Geometry check sheet. Reference: the model listing, model coordinates, mm. Coordinates: 2 decimals unless noted, no trailing zeros. Loops run counter-clockwise (first coordinate to the right, second up) from the corner with the lowest first, then second, coordinate; pieces in that order, holes last.
Autodesk Inventor part; units mm, degrees
ref_plane "YZ Plane" through (0, 0, 0) normal (1, 0, 0) x (0, 1, 0)
ref_plane "XZ Plane" through (0, 0, 0) normal (0, 1, 0) x (-1, 0, 0)
ref_plane "XY Plane" through (0, 0, 0) normal (0, 0, 1) x (1, 0, 0)
ref_plane "Work Plane1" through (0, 0, 0) normal (0, 0, 1) x (1, 0, 0)
sketch "Sketch1" plane through (0, 0, 0) normal (0, 0, 1) x (1, 0, 0)
  circle A0 centre (-16.4512, 11.8299) radius 1.45
  circle A1 centre (-37.2, 11.8299) radius 1.45
  line L0 (-41.2012, 5.1624) -> (-41.2012, -2.0876)
  line L1 (-41.2012, -2.0876) -> (-38.2, -2.0876)
  line L2 (-38.2, -2.0876) -> (-38.2, -7.0876)
  line L3 (-38.2, -7.0876) -> (-41.2, -7.0876)
  line L4 (-41.2, -7.0876) -> (-41.2, -48.1342)
  line L5 (-41.2, -48.1342) -> (-20.7938, -54.7646)
  line L6 (-20.7938, -54.7646) -> (28.3237, 8.1029)
  line L7 (28.3237, 8.1029) -> (54.2162, 8.1029)
  line L8 (54.2162, 8.1029) -> (54.2162, 31.454)
  line L9 (54.2162, 31.454) -> (27.1735, 40.2407)
  line L10 (27.1735, 40.2407) -> (-12.4512, -10.4765)
  line L11 (-12.4512, -10.4765) -> (-12.4512, 5.6624)
  line L12 (-12.4512, 5.6624) -> (-15.7012, 5.6624)
  line L13 (-15.7012, 5.6624) -> (-15.7012, 8.1624)
  line L14 (-15.7012, 8.1624) -> (-12.4512, 8.1624)
  line L15 (-12.4512, 8.1624) -> (-12.4512, 32.1624)
  line L16 (-31.5338, 32.1624) -> (-41.2, 32.1624)
  line L17 (-41.2, 32.1624) -> (-41.2, 8.1624)
  line L18 (-41.2, 8.1624) -> (-38.2, 8.1624)
  line L19 (-38.2, 8.1624) -> (-38.2, 5.6624)
  line L20 (-38.2, 5.6624) -> (-41.2, 5.6624)
  line L21 (-41.2, 5.6624) -> (-41.2, 5.1624)
  line L22 (-41.2, 5.1624) -> (-41.2012, 5.1624)
  line L23 (-12.7012, -2.0876) -> (-12.7012, -7.0876)
  line L24 (-12.7012, -7.0876) -> (-15.7012, -7.0876)
  line L25 (-15.7012, -7.0876) -> (-15.7012, -2.0876)
  line L26 (-15.7012, -2.0876) -> (-12.7012, -2.0876)
  line L27 (-16.239, -63.6047) -> (29.7869, 5.1029)
  line L28 (29.7869, 5.1029) -> (60.3683, 5.1029)
  line L29 (60.3683, 5.1029) -> (60.3683, 31.9539)
  line L30 (60.3683, 31.9539) -> (57.3683, 35.6787)
  line L31 (57.3683, 35.6787) -> (27.4078, 45.4135)
  line L32 (27.4078, 45.4135) -> (-9.4512, -1.7639)
  line L33 (-9.4512, -1.7639) -> (-9.4512, 35.1624)
  line L34 (-9.4512, 35.1624) -> (-42.2, 35.1624)
  line L35 (-42.2, 35.1624) -> (-44.2, 35.1624)
  line L36 (-44.2, 35.1624) -> (-44.2, -54.5196)
  line L37 (-44.2, -54.5196) -> (-16.239, -63.6047)
  line L38 (-41.2, 5.1624) -> (-41.2, 5.6624)
  line L39 (-41.2, 5.6624) -> (-38.2, 5.6624)
  line L40 (-38.2, 5.6624) -> (-38.2, 8.1624)
  line L41 (-38.2, 8.1624) -> (-41.2, 8.1624)
  line L42 (-41.2, 8.1624) -> (-41.2, 32.1624)
  line L43 (-41.2, 32.1624) -> (-12.4512, 32.1624)
  line L44 (-12.4512, 32.1624) -> (-12.4512, 8.1624)
  line L45 (-12.4512, 8.1624) -> (-15.7012, 8.1624)
  line L46 (-15.7012, 8.1624) -> (-15.7012, 5.6624)
  line L47 (-15.7012, 5.6624) -> (-12.4512, 5.6624)
  line L48 (-12.4512, 5.6624) -> (-12.4512, -10.4765)
  line L49 (-12.4512, -10.4765) -> (27.1735, 40.2407)
  line L50 (27.1735, 40.2407) -> (54.2162, 31.454)
  line L51 (54.2162, 31.454) -> (54.2162, 8.1029)
  line L52 (54.2162, 8.1029) -> (28.3237, 8.1029)
  line L53 (28.3237, 8.1029) -> (-20.7938, -54.7646)
  line L54 (-20.7938, -54.7646) -> (-41.2, -48.1342)
  line L55 (-41.2, -48.1342) -> (-41.2, -7.0876)
  line L56 (-41.2, -7.0876) -> (-38.2, -7.0876)
  line L57 (-38.2, -7.0876) -> (-38.2, -2.0876)
  line L58 (-38.2, -2.0876) -> (-41.2012, -2.0876)
  line L59 (-41.2012, -2.0876) -> (-41.2012, 5.1624)
  line L60 (-41.2012, 5.1624) -> (-41.2, 5.1624)
  circle A2 centre (43.9499, 17.9141) radius 1.4
  circle A3 centre (43.9499, 30.4141) radius 1.4
  line L61 (-31.5338, 25.1624) -> (-31.5338, 32.1624)
  line L62 (-12.4512, 32.1624) -> (-22.3686, 32.1624)
  line L63 (-22.3686, 32.1624) -> (-22.3686, 25.1624)
  line L64 (-22.3686, 25.1624) -> (-31.5338, 25.1624)
extrude "Extrusion1" add sketch "Sketch1" along normal blind 2 contours L21 L20 L19 L18 L17 L16 L61 L64 L63 L43 L15 L14 L13 L12 L11 L10 L9 L8 L7 L6 L5 L4 L3 L2 L1 L0 | L43 L63 L64 L61 | L23 L24 L25 L26 | L37 L36 L35 L34 L33 L32 L31 L30 L29 L28 L27 | A2 | A3
sketch "Sketch4" plane through (0, 0, 2) normal (0, 0, 1) x (1, 0, 0)
  line L0 (-12.4512, -7.0876) -> (-12.4512, -15.0876)
  line L1 (-12.4512, -15.0876) -> (-41.2, -15.0876)
  line L2 (-41.2, -15.0876) -> (-41.2, -7.0876)
  line L3 (-41.2, -7.0876) -> (-12.4512, -7.0876)
  line L4 (-41.4512, -2.0876) -> (-41.4512, 5.9124)
  line L5 (-41.4512, 5.9124) -> (-12.4512, 5.9124)
  line L6 (-12.4512, 5.9124) -> (-12.4512, -2.0876)
  line L7 (-12.4512, -2.0876) -> (-41.4512, -2.0876)
  line L8 (31.1264, -1.592) -> (36.5437, 2.1484)
  line L9 (36.5437, 2.1484) -> (37.0695, 3.5361)
  line L10 (37.0695, 3.5361) -> (60.3683, 9.779)
  line L11 (60.3683, 9.779) -> (60.3683, 9.784)
  line L12 (60.3683, 9.784) -> (60.3683, 31.9539)
  line L13 (60.3683, 31.9539) -> (57.3683, 35.9287)
  line L14 (57.3683, 35.9287) -> (27.5635, 45.6128)
  line L15 (27.5635, 45.6128) -> (-9.4512, -1.7639)
  line L16 (-9.4512, -1.7639) -> (-9.4512, 35.4124)
  line L17 (-9.4512, 35.4124) -> (-44.2, 35.4124)
  line L18 (-44.2, 35.4124) -> (-44.2, -54.5196)
  line L19 (-44.2, -54.5196) -> (-16.239, -63.6047)
  line L20 (-16.239, -63.6047) -> (12.0348, -27.416)
  line L21 (12.0348, -27.416) -> (25.8734, -27.416)
  line L22 (25.8734, -27.416) -> (25.8734, -22.5432)
  line L23 (25.8734, -22.5432) -> (22.8734, -22.5432)
  line L24 (22.8734, -22.5432) -> (22.8734, -13.5432)
  line L25 (22.8734, -13.5432) -> (25.8734, -13.5432)
  line L26 (25.8734, -13.5432) -> (25.8734, 0.5361)
  line L27 (25.8734, 0.5361) -> (29.5751, 0.5361)
  line L28 (29.5751, 0.5361) -> (29.5751, -1.592)
  line L29 (29.5751, -1.592) -> (31.1264, -1.592)
  line L30 (-41.6, -6.6876) -> (-41.6, -15.4876)
  line L31 (-41.6, -15.4876) -> (-12.0512, -15.4876)
  line L32 (-12.0512, -15.4876) -> (-12.0512, -6.6876)
  line L33 (-12.0512, -6.6876) -> (-41.6, -6.6876)
  line L34 (-41.8512, 6.3124) -> (-41.8512, -2.4876)
  line L35 (-41.8512, -2.4876) -> (-12.0512, -2.4876)
  line L36 (-12.0512, -2.4876) -> (-12.0512, 6.3124)
  line L37 (-12.0512, 6.3124) -> (-41.8512, 6.3124)
  point P0 (0, 0)
  dimension "d13" = 0.4
  dimension "d14" = 0.4
extrude "Extrusion4" cut sketch "Sketch4" against normal through all contours L0 L1 L2 L3 | L4 L5 L6 L7 | L33 L32 L31 L30 | L37 L36 L35 L34
properties part number "cellSTORM_v5_microscope_cover"
(1) Sectioned sample at D-D on y = -31. Record the cut outline in (x, z).
Findings:
outline: (-44.2, 0) - (5.6, 0) - (5.6, 2) - (-44.2, 2) - close
(2) Scan lines: L1, parallel to X at y = 1.5, z = 1.6; L2, parallel to X at y = 4, z = 1.6; L3, parallel to Y at x = -37.2, z = 1.6. Record each from-to range of solid material in increasing order.
Findings:
L1: x = -44.2 to -41.85, -12.05 to -9.45, -6.9 to 27.37
L2: x = -44.2 to -41.85, -12.05 to -9.45, -4.95 to 29.05
L3: y = -56.79 to -15.49, -6.69 to -2.49, 6.31 to 10.38, 13.28 to 35.16
(3) Sectioned sample at C-C on x = 43. Record the cut outline in (y, z), and give its area (3 significant figures).
Findings:
outline: (5.1, 0) - (40.35, 0) - (40.35, 2) - (5.1, 2) - close
area: 70.5 mm2
(4) Gauge pin test, flat ends, axial feed: pin 1 Ø4 at (x, y) = (-16.45, 11.83) entering from -Z; pin 2 Ø1 at (y, z) = (3.5, 1) entering from +X; pin 3 Ø1 at (x, z) = (-21.5, 1) entering from +Y. Record the tip position at first contact, or that the pin passes through.
Findings:
pin 1: stops at z = 0
pin 2: stops at x = 29.05
pin 3: stops at y = 35.16
(5) Sectioned sample at B-B on z = 1.7. Record the cut outline in (x, y).
Findings:
outline: (-44.2, -54.52) - (-16.24, -63.6) - (29.79, 5.1) - (60.37, 5.1) - (60.37, 31.95) - (57.37, 35.68) - (27.41, 45.41) - (-9.45, -1.76) - (-9.45, 35.16) - (-44.2, 35.16) - close; hole (-41.85, -2.49) - (-12.05, -2.49) - (-12.05, 6.31) - (-41.85, 6.31) - close; hole (-41.6, -15.49) - (-12.05, -15.49) - (-12.05, -6.69) - (-41.6, -6.69) - close; hole circle Ø2.9 at (-37.2, 11.83); hole circle Ø2.9 at (-16.45, 11.83)
(6) Sectioned sample at A-A on x = -37.2. Record the cut outline in (y, z).
Findings:
outline: (-56.79, 0) - (-15.49, 0) - (-15.49, 2) - (-56.79, 2) - close; (-6.69, 0) - (-2.49, 0) - (-2.49, 2) - (-6.69, 2) - close; (6.31, 0) - (10.38, 0) - (10.38, 2) - (6.31, 2) - close; (13.28, 0) - (35.16, 0) - (35.16, 2) - (13.28, 2) - close
(7) Draft check along Y on faces 1 (the flat face through (-30.415, -58.999, 0.986)), 2 (the flat face through (9.24, 22.16, 0.99)), 3 (the cylindrical face through (-38.27, 10.85, 0.99)). Enter one of: +Y half, -Y half, draft (parallel to the pull), parting line (faces both ways), or undercut.
Findings:
face 1: -Y half
face 2: +Y half
face 3: undercut
